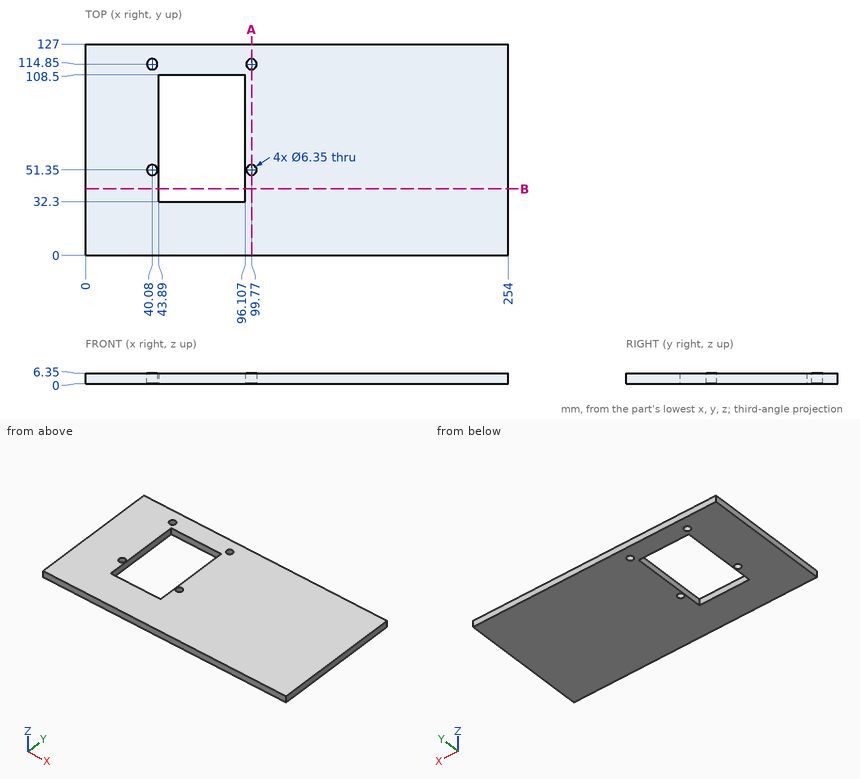
The drawing under review shows one solid part. Ordinate dimensions are in mm from its lowest x, y, z. Round coordinates to 2 decimals unless told otherwise and drop trailing zeros. Loops run counter-clockwise (first coordinate to the right, second up) from the corner with the lowest first, then second, coordinate; pieces in that order, holes last. Notation, with made-up numbers: (45, 13.25) -> (65, 13.25) arc R20 cw to (65, 38.25) -> close; hole circle Ø5 at (76.5, 22.25). An arc over 180 degrees is marked (long way). One line per question, with ' | ' between items. Start each with the question number.
Item 1: Add section A-A, the plane x = 99.77. Count the separate pieces of the cut face and the enclosed holes in it, then the cut area to 3 significant figures.
Item 2: Add section B-B, the plane y = 40. Write out the cut boundary in (x, z).
Item 3: Wall thickness on line 1 along Y through (x, z) = (99.77, 3.5) (1 decimal); line 2 along X through (y, z) = (93, 5.75); line 3 along Y through (x, z) = (47.5, 1): over which ranges is each line inside the solid? List them lowest first. Write a range as [from, to].
Item 4: For pin 1 (5.5 mm diameter, centred on x = 40.08, y = 114.85, fed in from +Z), flat-tipped, find the tip position at first contact; note if it passes through.
Return value:
1) separate pieces: 3 | enclosed holes: 0 | area: 726 mm2
2) outline: (0, 0) -> (43.89, 0) -> (43.89, 6.35) -> (0, 6.35) -> close; (96.11, 0) -> (254, 0) -> (254, 6.35) -> (96.11, 6.35) -> close
3) line 1: y = [0, 48.2], [54.5, 111.7], [118, 127] | line 2: x = [0, 43.89], [96.11, 254] | line 3: y = [0, 32.3], [108.5, 127]
4) pin 1: passes through
